Verification items for the finished model (mm, model axes). A direction names the side the tool comes from. Round coordinates to 2 decimals unless told otherwise and drop trailing zeros. Order: outer loops, then holes, each group sorted by start corner. A loop starts at its lowest first (then second) coordinate and runs counter-clockwise, first axis right, second up. Notation, with made-up numbers: (-21, -5.5) -> (0, -5.5) arc R15 ccw to (0, 18.5) -> close; hole circle Ø4 at (35, 32). An arc over 180 degrees is marked (long way). Return JSON: item names as keys, results as strings. Group by question number.
Item 1: Depth check by flat-ended pin: pin 1 Ø10 at (y, z) = (7, 19) entering from +X; pin 2 Ø3 at (x, z) = (7, 3) entering from +Y; pin 3 Ø1 at (y, z) = (2, 12.5) entering from +X; pin 4 Ø8 at (y, z) = (-2, 10) entering from -X. Enter the tip coordinate at first touch or a pass-through.
Item 2: Scan lines: probe 1 along Y at (x, z) = (0, 12.75); probe 2 along X at (y, z) = (4, 19.5); probe 3 along Z at (x, y) = (2.75, -8.5). Record each from-to range of solid material in increasing order. Write a range as from..to.
Item 3: Access from +Z, -Z, +X, -X, +Y, -Y to the whole of each face (thin tool, end or side, straight path). Record for faces 1 (the flat face through (4, -2, 0)), 2 (the flat face through (-2, 2, 18)).
Item 4: Sectioned sample at A-A on x = 0. Record the cut outline in (y, z), plus the area to 3 significant figures.
Item 5: Draft check along X on faces 3 (the cylindrical face through (4.38, -8.43, 12.34)), 4 (the cylindrical face through (0.867, -3.905, 8.874)), 5 (the flat face through (2, -2, 25)). Enter one of: pulls with the +X half, pulls with the -X half, needs draft (parallel to the pull), parting line crosses it, or undercut.
Item 6: Sectioned sample at C-C on z = 9.25. Record the cut outline in (x, y), plus the area to 3 significant figures.
```python
from build123d import *

# Parameters (mm, degrees)
SKETCH_1_R          = 9.5
SKETCH_1_R_2        = 2.5
EXTRUDE_1_DEPTH     = 25
CHAMFER_1_SIZE      = 1
SKETCH_2_R          = 4
CUT_EXTRUDE_1_DEPTH = 18


with BuildPart() as part:
    # 草图1 → 凸台-拉伸1 (new body)
    with BuildSketch(Plane.XY):
        Circle(SKETCH_1_R)
        Circle(SKETCH_1_R_2, mode=Mode.SUBTRACT)
    extrude(amount=EXTRUDE_1_DEPTH)

    # 倒角1
    chamfer_1_edges = [part.edges().sort_by_distance(p)[0] for p in [
        (-9.5, 0, 0),
        (-9.5, 0, 25),
    ]]
    chamfer(chamfer_1_edges, length=CHAMFER_1_SIZE)

    # 草图2 → 切除-拉伸1 (cut)
    with BuildSketch(Plane(origin=(0, 0, 0), x_dir=(-1, 0, 0), z_dir=(0, 0, -1))):
        Circle(SKETCH_2_R)
    extrude(amount=-CUT_EXTRUDE_1_DEPTH, mode=Mode.SUBTRACT)


solid = part.part
```
Recorded:
{
 "1": {"pin 1": "x = 9.29", "pin 2": "y = 7.75", "pin 3": "x = 9.38", "pin 4": "x = -9.5"},
 "2": {"probe 1": "-9.5..-4, 4..9.5", "probe 2": "-8.62..8.62", "probe 3": "0.43..24.57"},
 "3": {"face 1": "-Z, +X, -X, +Y, -Y", "face 2": "-Z"},
 "4": {"outline": "(-9.5, 1) -> (-8.5, 0) -> (-4, 0) -> (-4, 18) -> (-2.5, 18) -> (-2.5, 25) -> (-8.5, 25) -> (-9.5, 24) -> close; (2.5, 18) -> (4, 18) -> (4, 0) -> (8.5, 0) -> (9.5, 1) -> (9.5, 24) -> (8.5, 25) -> (2.5, 25) -> close", "area": "294 mm²"},
 "5": {"face 3": "parting line crosses it", "face 4": "undercut", "face 5": "needs draft"},
 "6": {"outline": "circle Ø19 at (0, 0); hole circle Ø8 at (0, 0)", "area": "233 mm²"}
}
